Autodesk Inventor part; units mm, degrees
ref_plane "FDT_MOUNT_XY" through (0, -14.2, 0) normal (0, 1, 0) x (-1, 0, 0)
ref_plane "FDT_MOUNT_YZ" through (0, -14.2, 0) normal (-1, 0, 0) x (0, 0, 1)
ref_plane "FDT_MOUNT_ZX" through (0, -14.2, 0) normal (0, 0, 1) x (0, 1, 0)
sketch "Sketch_14" plane through (0, 0, 0) normal (1, 0, 0) x (0, 1, 0)
  line L0 (-19.25, 0) -> (12.3, 0)
  line L1 (12.3, 0) -> (12.3, -2.19)
  line L2 (12.3, -2.19) -> (10.7, -3.15)
  line L3 (10.7, -3.15) -> (11.77, -3.15)
  line L4 (11.77, -3.15) -> (12.3, -3.3971)
  line L5 (12.3, -3.3971) -> (12.3, -3.55)
  line L6 (12.3, -3.55) -> (12.1, -3.75)
  line L7 (12.1, -3.75) -> (10.7, -3.75)
  line L8 (10.7, -3.75) -> (10.7, -5.75)
  line L9 (10.7, -5.75) -> (10.1515, -6.7)
  line L10 (10.1515, -6.7) -> (4.2, -6.7)
  line L11 (4.2, -6.7) -> (4.2, -6.9)
  line L12 (4.2, -6.9) -> (-11.5, -6.9)
  line L13 (-11.5, -6.9) -> (-11.5, -6.075)
  arc A0 (-11.5, -6.075) -> (-11.8, -6.375) centre (-11.5, -6.375) ccw
  line L14 (-11.8, -6.375) -> (-11.8, -6.75)
  line L15 (-11.8, -6.75) -> (-12.6, -6.75)
  line L16 (-12.6, -6.75) -> (-12.6, -6.575)
  line L17 (-12.6, -6.575) -> (-14.2, -6.575)
  line L18 (-14.2, -6.575) -> (-14.2, -4.864)
  line L19 (-14.2, -4.864) -> (-18.669, -4.864)
  line L20 (-18.669, -4.864) -> (-19.25, -4.283)
  line L21 (-19.25, -4.283) -> (-19.25, 0)
  line L22 (-19.25, 0) -> (12.3, 0)
revolve "Revolution1" add sketch "Sketch_14" angle 360 about axis through (0, -19.25, 0) along (0, -1, 0)
thread "Thread1"
sketch "Sketch_15" plane through (0, 12.3, 0) normal (0, 1, 0) x (1, 0, 0)
  line L0 (-12, -6.9282) -> (0, -13.8564)
  line L1 (0, -13.8564) -> (12, -6.9282)
  line L2 (12, -6.9282) -> (12, 6.9282)
  line L3 (12, 6.9282) -> (0, 13.8564)
  line L4 (0, 13.8564) -> (-12, 6.9282)
  line L5 (-12, 6.9282) -> (-12, -6.9282)
  line L6 (-6, -3.4641) -> (0, -6.9282)
  line L7 (0, -6.9282) -> (6, -3.4641)
  line L8 (6, -3.4641) -> (6, 3.4641)
  line L9 (6, 3.4641) -> (0, 6.9282)
  line L10 (0, 6.9282) -> (-6, 3.4641)
  line L11 (-6, 3.4641) -> (-6, -3.4641)
extrude "Extrusion1" cut sketch "Sketch_15" against normal blind 6.6
sketch "Sketch_16" plane through (0, 12.3, 0) normal (0, 1, 0) x (1, 0, 0)
  line L0 (-0.4, 3.0237) -> (-0.4, -3.0237)
  arc A0 (-0.4, -3.0237) -> (0.4, -3.0237) centre (0, 0) ccw
  line L1 (0.4, -3.0237) -> (0.4, 3.0237)
  arc A1 (0.4, 3.0237) -> (-0.4, 3.0237) centre (0, 0) ccw
extrude "Extrusion2" cut sketch "Sketch_16" against normal blind 1.2
sketch "Sketch_11" plane through (0, 0, 0) normal (1, 0, 0) x (0, 1, 0)
  line L0 (0, 0) -> (0, 22.5)
  line L1 (0, 22.5) -> (2.3, 22.5)
  line L2 (2.3, 22.5) -> (4.7847, 22.0619)
  arc A0 (4.95, 21.8649) -> (4.7847, 22.0619) centre (4.75, 21.8649) ccw
  line L3 (4.95, 21.8649) -> (4.95, 21)
  line L4 (4.95, 21) -> (3.1, 21)
  arc A1 (3.1, 21) -> (2.7, 20.6) centre (3.1, 20.6) ccw
  line L5 (2.7, 20.6) -> (2.7, 20)
  line L6 (2.7, 20) -> (3.55, 20)
  line L7 (3.55, 20) -> (3.75, 19.8)
  line L8 (3.75, 19.8) -> (3.75, 18.6)
  line L9 (3.75, 18.6) -> (4.85, 18.6)
  line L10 (4.85, 18.6) -> (4.85, 17.1)
  line L11 (4.85, 17.1) -> (5.1, 16.667)
  line L12 (5.1, 16.667) -> (5.1, 9.5)
  line L13 (5.1, 9.5) -> (3.6, 8)
  line L14 (3.6, 8) -> (3.6, 0)
  line L15 (3.6, 0) -> (0, 0)
  line L16 (0, 0) -> (0, 22.5)
revolve "Revolution2" add sketch "Sketch_11" angle 360 about axis through (0, 0, 0) along (0, 0, -1)
sketch "Sketch_17" plane through (0, 0, 0) normal (1, 0, 0) x (0, 1, 0)
  line L0 (0, 0) -> (0, 22.5)
  line L1 (0, 22.5) -> (2.3, 22.5)
  line L2 (2.3, 22.5) -> (4.7847, 22.0619)
  arc A0 (4.95, 21.8649) -> (4.7847, 22.0619) centre (4.75, 21.8649) ccw
  line L3 (4.95, 21.8649) -> (4.95, 21)
  line L4 (4.95, 21) -> (3.1, 21)
  arc A1 (3.1, 21) -> (2.7, 20.6) centre (3.1, 20.6) ccw
  line L5 (2.7, 20.6) -> (2.7, 20.085)
  line L6 (2.7, 20.085) -> (3.55, 20.085)
  line L7 (3.55, 20.085) -> (3.75, 19.885)
  line L8 (3.75, 19.885) -> (3.75, 18.6)
  line L9 (3.75, 18.6) -> (4.85, 18.6)
  line L10 (4.85, 18.6) -> (4.85, 17.1)
  line L11 (4.85, 17.1) -> (5.1, 16.667)
  line L12 (5.1, 16.667) -> (5.1, 9.5)
  line L13 (5.1, 9.5) -> (3.6, 8)
  line L14 (3.6, 8) -> (3.6, 0)
  line L15 (3.6, 0) -> (0, 0)
  line L16 (0, 0) -> (0, 22.5)
revolve "Revolution3" add sketch "Sketch_17" angle 360 about axis through (0, 0, 0) along (0, 0, -1)
sketch "Sketch_18" plane through (0, 0, 0) normal (0, 0, 1) x (1, 0, 0)
  arc A0 (-3.8158, 1.5) -> (-3.8158, -1.5) centre (0, 0) ccw
  line L0 (-3.8158, -1.5) -> (3.8158, -1.5)
  arc A1 (3.8158, -1.5) -> (3.8158, 1.5) centre (0, 0) ccw
  line L1 (3.8158, 1.5) -> (-3.8158, 1.5)
extrude "Extrusion3" add sketch "Sketch_18" along normal blind 11.25
sketch "Sketch_5" plane through (0, 0, 0) normal (1, 0, 0) x (0, 1, 0)
  line L0 (0, 0) -> (0, 22.5)
  line L1 (0, 22.5) -> (2.3, 22.5)
  arc A0 (2.3, 22.5) -> (2, 22.2) centre (2.3, 22.2) ccw
  line L2 (2, 22.2) -> (2, 7.5)
  line L3 (2, 7.5) -> (1, 7.5)
  line L4 (1, 7.5) -> (1, 0)
  line L5 (1, 0) -> (0, 0)
  line L6 (0, 0) -> (0, 22.5)
revolve "Revolution4" cut sketch "Sketch_5" angle 360 about axis through (0, 0, 0) along (0, 0, -1)
sketch "Sketch8" plane through (0, -19.25, 0) normal (0, -1, 0) x (1, 0, 0)
  point P0 (0, 0)
hole "Hole1" at (0, -19.25, 0) direction (0, 1, 0) diameter 3 depth 21.25 countersink diameter 3.3464 countersink angle 60
ref_plane "FDT_MOUNT_XY" through (0, -14.2, 0) normal (0, 1, 0) x (-1, 0, 0)
ref_plane "FDT_MOUNT_YZ" through (0, -14.2, 0) normal (-1, 0, 0) x (0, 0, 1)
ref_plane "FDT_MOUNT_ZX" through (0, -14.2, 0) normal (0, 0, 1) x (0, 1, 0)
ref_plane "FDT_SCHLAUCH_XY" through (0, 0, 7.5) normal (0, 0, 1) x (1, 0, 0)
ref_plane "FDT_SCHLAUCH_YZ" through (0, 0, 7.5) normal (1, 0, 0) x (0, 1, 0)
ref_plane "FDT_SCHLAUCH_ZX" through (0, 0, 7.5) normal (0, 1, 0) x (0, 0, 1)
ref_plane "Zylinder_XY" through (0, -19.25, 0) normal (0, 1, 0) x (1, 0, 0)
ref_plane "Zylinder_YZ" through (0, -19.25, 0) normal (1, 0, 0) x (0, 0, -1)
ref_plane "Zylinder_ZX" through (0, -19.25, 0) normal (0, 0, -1) x (0, 1, 0)
ref_plane "anbau_XY" through (0, -14.2, 0) normal (0, 1, 0) x (1, 0, 0)
ref_plane "anbau_YZ" through (0, -14.2, 0) normal (1, 0, 0) x (0, 0, -1)
ref_plane "anbau_ZX" through (0, -14.2, 0) normal (0, 0, -1) x (0, 1, 0)
properties part number "193143 GRLA-1/8-QS-4-D"
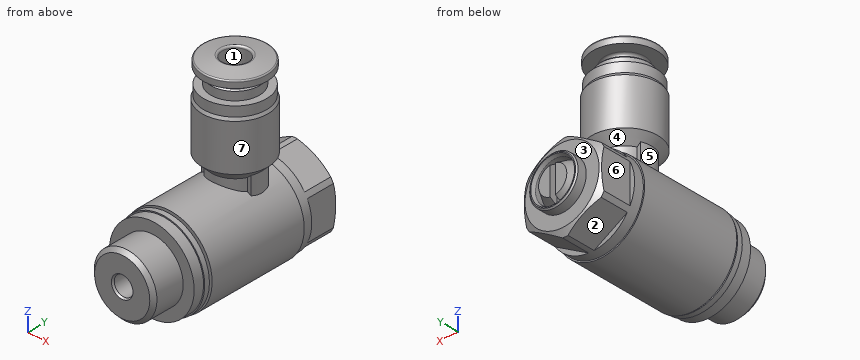
Build history of the part. All positions in model axes, mm. Face numbers are marked on the shaded views. A direction names the side the tool comes from. Give positions to 0.01 mm unless a question says otherwise; leave off trailing zeros. One line per question, with ' | ' between items. Start each with the question number.
1) Probe L1, parallel to X at y = -5.25, z = 0; L2, parallel to X at y = 0, z = 15.25; L3, parallel to Y at x = -5.5, z = 0.25. List the from-to ranges inside material, lowest first.
2) 3-axis set-ups, long thin cutter, end or side, ignore diameter. For the marked faces 5, 6 and 7: which of +Z, -Z, +X, -X, +Y, -Y reach the whole face in a straight line?
3) Two-plate mould, pull along Y, no slides. Class the marked faces 1, 2, 3 and 4: released by +Y, released by -Y, zero draft, split by the parting line, or undercut.
4) Pin check, flat tips, straight feed: pin 1 (3.5 mm diameter, centred on x = -3, z = -5, fed in from +Y); pin 2 (0.6 mm diameter, centred on y = 11.5, z = -1, fed in from +X); pin 3 (0.6 mm diameter, centred on x = 0, z = 0, fed in from +Y); pin 4 (4 mm diameter, centred on x = -1, y = 3.5, fed in from -Z). Stop position of each tip, or through.
Return value:
1) L1: -6.9 to -1.5, 1.5 to 6.9 | L2: -5.1 to -2, 2 to 5.1 | L3: -14.2 to 10.7
2) face 5: -X | face 6: +Z, -Z, -X, +Y | face 7: +Z
3) face 1: undercut | face 2: zero draft | face 3: released by +Y | face 4: split by the parting line
4) pin 1: y = 10.7 | pin 2: x = 3.68 | pin 3: y = 11.1 | pin 4: z = -6.9
